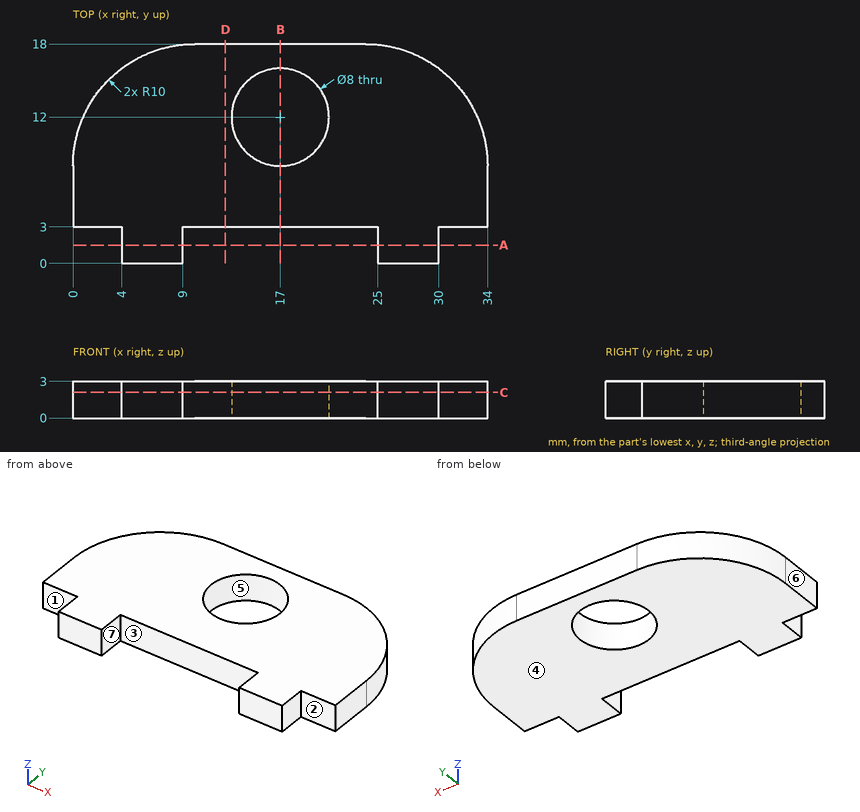
Input: dimensioned drawing with shaded views. Units: mm. Origin: part minimum x, y, z. A direction names the side the tool comes from. Coordinates: 2 decimals unless noted, no trailing zeros. Order: outer loops, then holes, each group sorted by start corner. A loop starts at its lowest first (then second) coordinate and runs counter-clockwise, first axis right, second up.
1. Draft query along X for the marked faces 4, 5, 6 and 7. Return one class per face: +X half, -X half, draft (parallel to the pull), parting line (faces both ways), or undercut.
Checked values:
face 4: draft
face 5: undercut
face 6: -X half
face 7: undercut
2. Ray query, line 1 along X through (y, z) = (1, 2.35); line 2 along Y through (x, z) = (17, 1.65); line 3 along X through (y, z) = (9.25, 0.7). Return the intervals inside material, ascending.
Checked values:
line 1: x = 4 to 9, 25 to 30
line 2: y = 3 to 8, 16 to 18
line 3: x = 0.08 to 14.1, 19.9 to 33.92
3. Cut plane D-D, the plane x = 12.5. Return loops of the section in (y, z), plus the area to 3 significant figures.
Checked values:
outline: (3, 0) - (18, 0) - (18, 3) - (3, 3) - close
area: 45.0 mm2
4. Access query for the marked faces 1, 2 and 3. Directions: +Z, -Z, +X, -X, +Y, -Y. A direction counts if a zero-diameter tool reaches every point of the face in a straight line with its end or side. Return the directions, or none.
Checked values:
face 1: +Z, -Z, -X, -Y
face 2: +Z, -Z, +X, -Y
face 3: +Z, -Z, -Y
5. Cut plane B-B, the plane x = 17. Return loops of the section in (y, z).
Checked values:
outline: (3, 0) - (8, 0) - (8, 3) - (3, 3) - close; (16, 0) - (18, 0) - (18, 3) - (16, 3) - close
6. Cut plane A-A, the plane y = 1.5. Return loops of the section in (x, z).
Checked values:
outline: (4, 0) - (9, 0) - (9, 3) - (4, 3) - close; (25, 0) - (30, 0) - (30, 3) - (25, 3) - close
7. Cut plane C-C, the plane z = 2.1. Return loops of the section in (x, y).
Checked values:
outline: (0, 3) - (4, 3) - (4, 0) - (9, 0) - (9, 3) - (25, 3) - (25, 0) - (30, 0) - (30, 3) - (34, 3) - (34, 8) arc R10 ccw to (24, 18) - (10, 18) arc R10 ccw to (0, 8) - close; hole circle Ø8 at (17, 12)
8. Contact query for flat-ended pins moving along their axis: P1, Ø1.5, axis at y = 1, z = 2, coming from the +X side; P2, Ø10.5, axis at x = 17, y = 12, coming from the +Z side; P3, Ø1.5, axis at y = 1, z = 1, coming from the -X side. Output: stop coordinate, or through.
Checked values:
P1: stops at x = 30
P2: stops at z = 3
P3: stops at x = 4
